from build123d import *

# Parameters (mm, degrees)
SKETCH1_R               = 7.112
BOSS_EXTRUDE1_DEPTH     = 33.02
SKETCH2_OUTSIDE_W       = 23.956
SKETCH2_OUTSIDE_H       = 23.956
SKETCH2_OUTSIDE_R       = 4.6355
CUT_EXTRUDE1_DEPTH      = 29.6926
CUT_EXTRUDE2_DEPTH      = 35.517843038
CUT_EXTRUDE2_DEPTH_BACK = 35.517843038
SKETCH3_R               = 1.905
BOSS_EXTRUDE2_DEPTH     = 0.254
FILLET1_R               = 0.2286
FILLET2_R               = 0.635


with BuildPart() as part:
    # Sketch1 → Boss-Extrude1 (new body)
    with BuildSketch(Plane(origin=(0, 0, 0), x_dir=(1, 0, 0), z_dir=(0, 1, 0))):
        with Locations(Location((0, 0, 0), (0, 0, 270))):
            Circle(SKETCH1_R)
    extrude(amount=BOSS_EXTRUDE1_DEPTH)

    # Sketch2 outside → Cut-Extrude1 (cut)
    with BuildSketch(Plane(origin=(0, 33.02, 0), x_dir=(1, 0, 0), z_dir=(0, 1, 0))):
        Rectangle(SKETCH2_OUTSIDE_W, SKETCH2_OUTSIDE_H)
        with Locations(Location((0, 0, 0), (0, 0, 270))):
            Circle(SKETCH2_OUTSIDE_R, mode=Mode.SUBTRACT)
    extrude(amount=-CUT_EXTRUDE1_DEPTH, mode=Mode.SUBTRACT)

    # Sketch3 → Cut-Extrude2 (cut, two sides: drawn at the far end of the back side and taken through both)
    with BuildSketch(Plane(origin=(0, 0, 0), x_dir=(0, 0, -1), z_dir=(1, 0, 0)).offset(-CUT_EXTRUDE2_DEPTH_BACK)):
        with Locations((0, 27.9908)):
            Circle(SKETCH3_R)
    extrude(amount=CUT_EXTRUDE2_DEPTH + CUT_EXTRUDE2_DEPTH_BACK, mode=Mode.SUBTRACT)

    # Sketch4 → Boss-Extrude2 (add)
    # profile 1 of 2: a face of its own
    with BuildSketch(Plane.XZ):
        Polygon((-1.505619488, 2.477183377), (0.109765127, -1.022816623), (-0.231681187, -1.022816623), (-0.749109071, 0.098978249), (-2.335747693, 0.098978249), (-2.867899135, -1.022816623), (-3.210747693, -1.022816623), (-1.550491283, 2.477183377), align=None)
        Polygon((-1.531560994, 1.794991871), (-2.165375097, 0.457952608), (-0.914573815, 0.457952608), align=None, mode=Mode.SUBTRACT)
    # profile 2 of 2: a face of its own
    with BuildSketch(Plane.XZ):
        Polygon((0.737970256, 2.477183377), (2.443098461, 2.477183377), (2.443098461, 2.118209018), (1.05207282, 2.118209018), (1.05207282, 1.041285942), (2.443098461, 1.041285942), (2.443098461, 0.682311583), (1.05207282, 0.682311583), (1.05207282, -1.022816623), (0.737970256, -1.022816623), align=None)
    extrude(amount=BOSS_EXTRUDE2_DEPTH)

    # Fillet1
    fillet1_edges = [part.edges().sort_by_distance(p)[0] for p in [
        (0, 0, -7.112),
        (0, 3.3274, -7.112),
    ]]
    fillet(fillet1_edges, radius=FILLET1_R)

    # Fillet2
    fillet2_edges = [part.edges().sort_by_distance(p)[0] for p in [
        (0, 33.02, -4.6355),
    ]]
    fillet(fillet2_edges, radius=FILLET2_R)


solid = part.part
For this review, take the finished solid that the model builds, in its own axes (mm). A direction names the side the tool comes from. Give positions to 0.01 mm unless a question says otherwise; leave off trailing zeros. Loops run counter-clockwise (first coordinate to the right, second up) from the corner with the lowest first, then second, coordinate; pieces in that order, holes last. Notation, with made-up numbers: M 39,58.5 L 72,58.5 A7 cw 72,68.5 Z; hole C 85.5,-8.5 d10. An arc over 180 degrees is marked long. Answer as a JSON object with one key per item and string values. Group by question number.
Q1. Insertion check: P1, Ø2, axis at y = 6.5, z = 0, coming from the -X side; P2, Ø2, axis at y = 19.5, z = -1, coming from the +X side; P3, Ø4, axis at y = 26, z = 4.5, coming from the -X side. Each pin has a flat end and moves straight along its axis. Give the tip position at first contact, or say it passes through.
Q2. Mouldability with a two-part tool opening along X and no side actions: class faces 3 (the flat face through (0, 33.02, 0)), 4 (the cylindrical face through (1.392, 18.06, 4.421)), 5 (the flat face through (-1.5, 0, 1)) as +X half, -X half, draft (parallel to the pull), parting line (faces both ways), or undercut.
Q3. For probe 1 along Y at (x, z) = (-0.75, 0); probe 2 along X at (y, z) = (8, 0.25); probe 3 along Y at (x, z) = (1.75, -5.5), list the stretches that pass through material, from the lowest coordinate up. Write a range as [from, to].
Q4. Tool access review of faces 1 (the flat face through (0, 3.327, -5)), 2 (the cylindrical face through (-6.943, 1.644, -1.542)): name each direction out of +Z, -Z, +X, -X, +Y, -Y from which nothing blocks a thin tool from reaching the whole face with its end or side.
Q5. Add section A-A on y = 12.5. Give the boundary of the cut face in (x, z), and give its area (3 significant figures).
Checked values:
{
 "1": {"P1": "x = -4.64", "P2": "x = 4.64", "P3": "x = -3.9"},
 "2": {"face 3": "draft", "face 4": "parting line", "face 5": "undercut"},
 "3": {"probe 1": "[0, 26.09], [29.9, 33.02]", "probe 2": "[-4.63, 4.63]", "probe 3": "[0, 3.33]"},
 "4": {"face 1": "+Y", "face 2": "+Y, -Y"},
 "5": {"outline": "C 0,0 d9.27", "area": "67.5 mm²"}
}
